```python
from build123d import *

# Parameters (mm, degrees)
F0_R     = 6.25
F1_DEPTH = 10
F1_TAPER = -20
F2_R     = 3.25
F3_DEPTH = 7.6
F6_R     = 44
F6_R_2   = 9.8897023427
F6_R_3   = 1.5
F7_DEPTH = 3
F8_R     = 4
F9_DEPTH = 25


with BuildPart() as f1:
    # F0 (on Top) → F1 (new body)
    with BuildSketch(Plane.XY):
        Circle(F0_R)
    extrude(amount=F1_DEPTH, taper=F1_TAPER)

    # F2 (on face) → F3 (cut)
    with BuildSketch(Plane(origin=(0, 0, 0), x_dir=(1, 0, 0), z_dir=(0, 0, -1))):
        Circle(F2_R)
    extrude(amount=-F3_DEPTH, mode=Mode.SUBTRACT)

    # F4 (on Front) → F5 (revolve, cut)
    with BuildSketch(Plane.XZ):
        with BuildLine():
            Line((0, 0), (0, 1.3641098567))
            ThreePointArc((0, 1.3641098567), (-3.198565917, 1.0191150111), (-6.25, 0))
            Line((-6.25, 0), (0, 0))
        make_face()
    revolve(axis=Axis((0, 0, -13.6358901433), (0, 0, -1)), mode=Mode.SUBTRACT)

    # F6 (on face) → F7 (join)
    with BuildSketch(Plane.XY.offset(10)):
        Circle(F6_R)
        with BuildLine():
            Line((-32.8414780938, -8.7998475335), (-14.4888873943, -3.8822856765))
            ThreePointArc((-14.4888873943, -3.8822856765), (-12.9903810568, -7.5), (-10.6066017178, -10.6066017178))
            Line((-10.6066017178, -10.6066017178), (-24.0416305603, -24.0416305603))
            ThreePointArc((-24.0416305603, -24.0416305603), (-29.4448637287, -17), (-32.8414780938, -8.7998475335))
        make_face(mode=Mode.SUBTRACT)
        with BuildLine():
            Line((-8.7998475335, -32.8414780938), (-3.8822856765, -14.4888873943))
            ThreePointArc((-3.8822856765, -14.4888873943), (0, -15), (3.8822856765, -14.4888873943))
            Line((3.8822856765, -14.4888873943), (8.7998475335, -32.8414780938))
            ThreePointArc((8.7998475335, -32.8414780938), (0, -34), (-8.7998475335, -32.8414780938))
        make_face(mode=Mode.SUBTRACT)
        with BuildLine():
            Line((24.0416305603, -24.0416305603), (10.6066017178, -10.6066017178))
            ThreePointArc((10.6066017178, -10.6066017178), (12.9903810568, -7.5), (14.4888873943, -3.8822856765))
            Line((14.4888873943, -3.8822856765), (32.8414780938, -8.7998475335))
            ThreePointArc((32.8414780938, -8.7998475335), (29.4448637287, -17), (24.0416305603, -24.0416305603))
        make_face(mode=Mode.SUBTRACT)
        with BuildLine():
            Line((-24.0416305603, 24.0416305603), (-10.6066017178, 10.6066017178))
            ThreePointArc((-10.6066017178, 10.6066017178), (-12.9903810568, 7.5), (-14.4888873943, 3.8822856765))
            Line((-14.4888873943, 3.8822856765), (-32.8414780938, 8.7998475335))
            ThreePointArc((-32.8414780938, 8.7998475335), (-29.4448637287, 17), (-24.0416305603, 24.0416305603))
        make_face(mode=Mode.SUBTRACT)
        Circle(F6_R_2, mode=Mode.SUBTRACT)
        with BuildLine():
            Line((32.8414780938, 8.7998475335), (14.4888873943, 3.8822856765))
            ThreePointArc((14.4888873943, 3.8822856765), (12.9903810568, 7.5), (10.6066017178, 10.6066017178))
            Line((10.6066017178, 10.6066017178), (24.0416305603, 24.0416305603))
            ThreePointArc((24.0416305603, 24.0416305603), (29.4448637287, 17), (32.8414780938, 8.7998475335))
        make_face(mode=Mode.SUBTRACT)
        with BuildLine():
            ThreePointArc((3.8822856765, 14.4888873943), (0, 15), (-3.8822856765, 14.4888873943))
            Line((-3.8822856765, 14.4888873943), (-8.7998475335, 32.8414780938))
            ThreePointArc((-8.7998475335, 32.8414780938), (0, 34), (8.7998475335, 32.8414780938))
            Line((8.7998475335, 32.8414780938), (3.8822856765, 14.4888873943))
        make_face(mode=Mode.SUBTRACT)
        Circle(F6_R_2)
        Circle(F6_R_3, mode=Mode.SUBTRACT)
    extrude(amount=F7_DEPTH)

    # F8
    f8_edges = [f1.edges().sort_by_distance(p)[0] for p in [
        (-9.889702, 0, 10),
        (-10.606602, -10.606602, 11.5),
        (-14.488887, -3.882286, 11.5),
        (-32.841478, -8.799848, 11.5),
        (-24.041631, -24.041631, 11.5),
        (8.799848, -32.841478, 11.5),
        (3.882286, -14.488887, 11.5),
        (-8.799848, 32.841478, 11.5),
        (-24.041631, 24.041631, 11.5),
        (-10.606602, 10.606602, 11.5),
        (32.841478, -8.799848, 11.5),
        (14.488887, -3.882286, 11.5),
        (10.606602, 10.606602, 11.5),
        (-3.882286, -14.488887, 11.5),
        (10.606602, -10.606602, 11.5),
        (24.041631, -24.041631, 11.5),
        (32.841478, 8.799848, 11.5),
        (14.488887, 3.882286, 11.5),
        (3.882286, 14.488887, 11.5),
        (-8.799848, -32.841478, 11.5),
        (-32.841478, 8.799848, 11.5),
        (-14.488887, 3.882286, 11.5),
        (-3.882286, 14.488887, 11.5),
        (8.799848, 32.841478, 11.5),
        (24.041631, 24.041631, 11.5),
    ]]
    fillet(f8_edges, radius=F8_R)

    # F9 (cut): a face of the model
    f9_faces = [f1.faces().sort_by_distance(p)[0] for p in [
        (0, 0, 10),
    ]]
    extrude(f9_faces, amount=-F9_DEPTH, mode=Mode.SUBTRACT)


solid = f1.part
```
The listing builds one solid part. Answer for the finished solid, in the listing's coordinates (mm). Round coordinates to 2 decimals unless told otherwise and drop trailing zeros. Write each loop counter-clockwise with the first axis right and the second up, starting at its lowest first coordinate (ties: lowest second). Pieces come first, ordered by that corner, then holes. Notation, with made-up numbers: (50, 55.25) -> (79, 55.25) arc R32 cw to (79, 82.25) -> close; hole circle Ø10 at (30, 15). An arc over 180 degrees is marked (long way). Answer as a JSON object with one key per item and string values. Group by question number.
Q1. Section C-C (z = 11.5) is taken. Count the separate pieces of the cut face and the enclosed holes in it, plus the area to 3 significant figures.
Q2. Section B-B (y = 27.5) is taken. Write down the section's boundary in (x, z), plus the area to 3 significant figures.
Q3. Section A-A (x = 20) is taken. Write down the section's boundary in (y, z), plus the area to 3 significant figures.
Q4. Determine the mould class of faces 1 (the face through (6.406, 2.017, 1.28)), 2 (the face through (9, 1, 13)), 3 (the face through (11.99, -10.77, 11.52)), 4 (the face through (31.295, 9.838, 11.521)) for opening direction Y: pulls with the +Y half, pulls with the -Y half, needs draft (parallel to the pull), parting line crosses it, or undercut.
Q5. Straight lines are drawn through the part: line 1 along Y through (x, z) = (3, 10.5); line 2 along Y through (x, z) = (-26, 12.5); line 3 along Z through (x, y) = (32, 14). For each, find the intervals that lie inside material, in ascending order.
Q6. Section D-D (z = 4.25) is taken. Write down the section's boundary in (x, y).
Q7. Each of these flat-tipped pins is pushed along its axis until it touches: pin 1 Ø3 at (x, z) = (-0.5, 9) entering from -Y; pin 2 Ø6 at (x, y) = (4.5, -23) entering from -Z; pin 3 Ø1.5 at (y, z) = (17.5, 9.5) entering from +X. Where does it stop, or does it pass through?
Check values:
{
 "1": {"separate pieces": "1", "enclosed holes": "7", "area": "4,690 mm^2"},
 "2": {"outline": "(-34.35, 10) -> (-7.37, 10) -> (-7.37, 13) -> (-34.35, 13) -> close; (7.37, 10) -> (34.35, 10) -> (34.35, 13) -> (7.37, 13) -> close", "area": "162 mm^2"},
 "3": {"outline": "(-39.19, 10) -> (-20, 10) -> (-20, 13) -> (-39.19, 13) -> close; (-5.36, 10) -> (5.36, 10) -> (5.36, 13) -> (-5.36, 13) -> close; (20, 10) -> (39.19, 10) -> (39.19, 13) -> (20, 13) -> close", "area": "147 mm^2"},
 "4": {"face 1": "parting line crosses it", "face 2": "needs draft", "face 3": "undercut", "face 4": "undercut"},
 "5": {"line 1": "-43.9 to -33.87, -15.55 to 15.55, 33.87 to 43.9", "line 2": "-35.5 to -21.57, -6.97 to 6.97, 21.57 to 35.5", "line 3": "10 to 13"},
 "6": {"outline": "circle Ø15.59 at (0, 0); hole circle Ø6.5 at (0, 0)"},
 "7": {"pin 1": "y = -44", "pin 2": "z = 10", "pin 3": "x = 40.61"}
}
